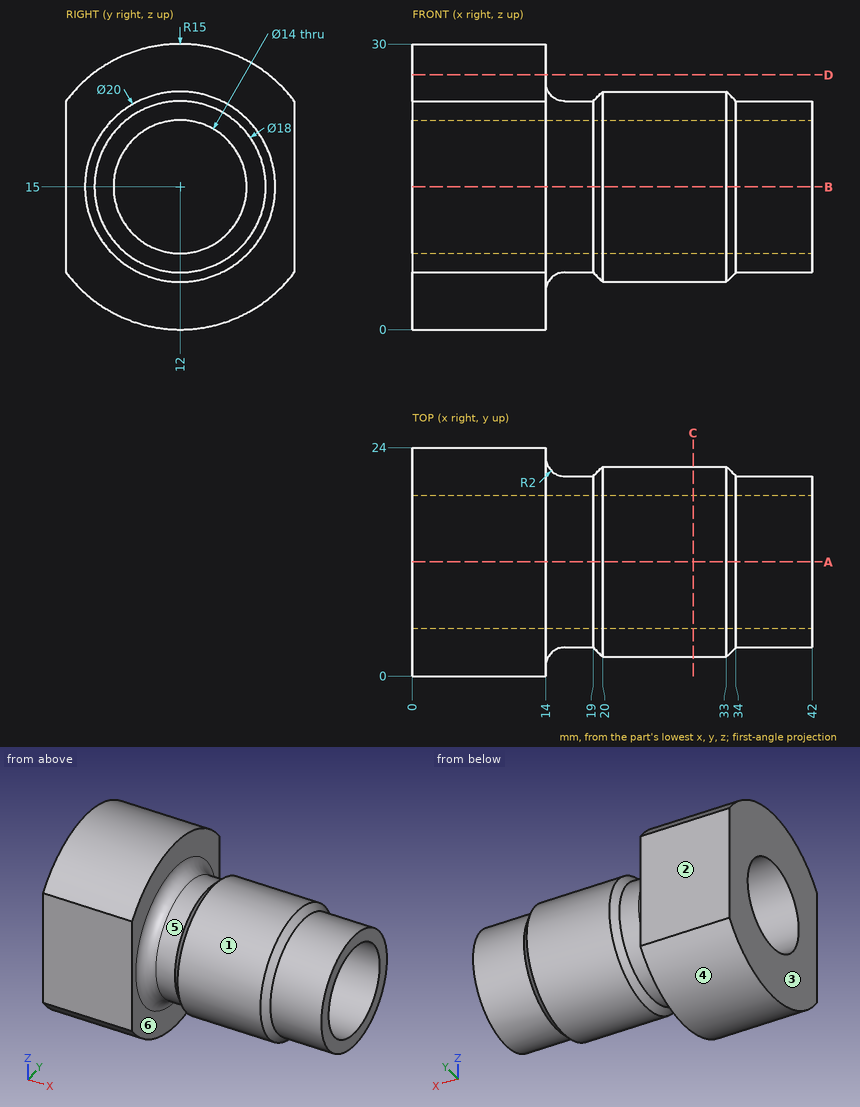
The figure shows three views and two pictorial views of one solid part (mm, origin at its lowest corner). Answer the questions. A direction names the side the tool comes from. Give positions to 0.01 mm unless a question says otherwise; leave off trailing zeros. Write each loop counter-clockwise with the first axis right and the second up, starting at its lowest first coordinate (ties: lowest second). Pieces come first, ordered by that corner, then holes.
Q1. For a pull along X with two mould halves and no side action, classify the marked faces 3, 4, 5 and 6 as released by +X, released by -X, zero draft, split by the parting line, or undercut.
Answer:
face 3: released by -X
face 4: zero draft
face 5: undercut
face 6: released by +X
Q2. Straight lines are drawn through the part: L1, parallel to Y at x = 10, z = 15; L2, parallel to X at y = 17.5, z = 24.75; L3, parallel to Y at x = 4.5, z = 19.5. For each, find the intervals that lie inside material, in ascending order.
Answer:
L1: y = 0 to 5, 19 to 24
L2: x = 0 to 14
L3: y = 0 to 6.64, 17.36 to 24
Q3. A tool of negligible diameter and unlimited length cuts with its end or side. For the marked faces 1 and 2, from which of +Z, -Z, +X, -X, +Y, -Y can it reach the whole face along a straight path? Write none if from no direction.
Answer:
face 1: +X
face 2: +Z, -Z, +X, -X, +Y
Q4. The part is cut by section B-B on z = 15. Give the vertices of the cut face in (x, y).
Answer:
outline: (0, 0) - (14, 0) - (14, 1) arc R2 cw to (16, 3) - (19, 3) - (20, 2) - (33, 2) - (34, 3) - (42, 3) - (42, 5) - (0, 5) - close; (0, 19) - (42, 19) - (42, 21) - (34, 21) - (33, 22) - (20, 22) - (19, 21) - (16, 21) arc R2 cw to (14, 23) - (14, 24) - (0, 24) - close
Q5. The part is cut by section C-C on x = 29.5. Give the vertices of the cut face in (y, z).
Answer:
outline: circle Ø20 at (12, 15); hole circle Ø14 at (12, 15)
Q6. The part is cut by section A-A on y = 12. Give the vertices of the cut face in (x, z), and give its area (3 significant figures).
Answer:
outline: (0, 0) - (14, 0) - (14, 4) arc R2 cw to (16, 6) - (19, 6) - (20, 5) - (33, 5) - (34, 6) - (42, 6) - (42, 8) - (0, 8) - close; (0, 22) - (42, 22) - (42, 24) - (34, 24) - (33, 25) - (20, 25) - (19, 24) - (16, 24) arc R2 cw to (14, 26) - (14, 30) - (0, 30) - close
area: 366 mm2
Q7. The part is cut by section D-D on z = 26.75. Give the vertices of the cut face in (x, y), and give its area (3 significant figures).
Answer:
outline: (0, 2.68) - (14, 2.68) - (14, 21.32) - (0, 21.32) - close
area: 261 mm2
Q8. Given pin 1 (12 mm diameter, centred on x = 27.5, y = 18, fed in from +Z); pin 2 (8 mm diameter, centred on x = 36.5, y = 7.5, fed in from -Z); pin 3 (1 mm diameter, centred on x = 31, z = 15, fed in from +Y), each flat-ended and moving along its own axis, determine where each tip first touches the part or whether it passes through.
Answer:
pin 1: stops at z = 25
pin 2: stops at z = 5.33
pin 3: stops at y = 22
